Autodesk Inventor part; units mm, degrees
ref_plane "YZ Plane" through (0, 0, 0) normal (1, 0, 0) x (0, 1, 0)
ref_plane "XZ Plane" through (0, 0, 0) normal (0, 1, 0) x (-1, 0, 0)
ref_plane "XY Plane" through (0, 0, 0) normal (0, 0, 1) x (1, 0, 0)
sketch "Szkic1" plane through (0, 0, 0) normal (0, 0, 1) x (1, 0, 0)
  line L0 (-10.5, 0) -> (0, 0)
  line L1 (0, 2) -> (-10.5, 2)
  line L2 (0, 2) -> (-5.359, -18)
  line L3 (-3.8837, -4.7669) -> (-2.0706, 2)
  line L4 (-3.8837, -4.7669) -> (-7.4295, -18)
  line L5 (-7.4295, -18) -> (-5.359, -18)
  dimension "d0" = 2
  dimension "d1" = 75
  dimension "d3" = 2
  dimension "d4" = 20
extrude "Wyciągnięcie proste1" add sketch "Szkic1" against normal blind 50
sketch "Szkic2" plane through (-5.359, -18, 0) normal (0.9659, -0.2588, 0) x (0, 0, -1)
  line L0 (42.7, 8.2894) -> (42.7, 10.6894)
  line L1 (38.3, 8.2894) -> (42.7, 8.2894)
  line L2 (7.3, 8.2894) -> (11.7, 8.2894)
  line L3 (11.7, 8.2894) -> (11.7, 10.6894)
  line L4 (42.7, 8.2894) -> (38.3, 8.2894)
  line L5 (38.3, 8.2894) -> (38.3, 10.6894)
  line L6 (38.3, 10.6894) -> (42.7, 10.6894)
  line L7 (42.7, 10.6894) -> (42.7, 8.2894)
  line L8 (11.7, 8.2894) -> (7.3, 8.2894)
  line L9 (7.3, 8.2894) -> (7.3, 10.6894)
  line L10 (7.3, 10.6894) -> (11.7, 10.6894)
  line L11 (11.7, 10.6894) -> (11.7, 8.2894)
  line L12 (43.7, 11.6894) -> (37.3, 11.6894)
  line L13 (37.3, 11.6894) -> (37.3, 7.2894)
  line L14 (37.3, 7.2894) -> (43.7, 7.2894)
  line L15 (43.7, 7.2894) -> (43.7, 11.6894)
  line L16 (12.7, 11.6894) -> (6.3, 11.6894)
  line L17 (6.3, 11.6894) -> (6.3, 7.2894)
  line L18 (6.3, 7.2894) -> (12.7, 7.2894)
  line L19 (12.7, 7.2894) -> (12.7, 11.6894)
  point P0 (0, 18.7737)
  dimension "d7" = 1
  dimension "d8" = 1
extrude "Wyciągnięcie proste2" cut sketch "Szkic2" against normal through all contours L1 L5 L6 L0 | L9 L10 L3 L2 | L15 L14 L13 L12 | L19 L18 L17 L16
sketch "Szkic3" plane through (0, 0, 0) normal (0, 0, 1) x (1, 0, 0)
  line L0 (-2.0706, 2) -> (-7.4295, -18)
  line L1 (-7.4295, -18) -> (-5.359, -18)
  line L2 (-5.359, -18) -> (0, 2)
  line L3 (0, 2) -> (-2.0706, 2)
  line L4 (-30.5, -19.37) -> (-8.3143, -19.37)
  line L5 (-7.4295, -18) -> (-8.3143, -19.37)
  line L6 (-8.3143, -19.37) -> (-5.7261, -19.37)
  line L7 (-5.7261, -19.37) -> (-5.359, -18)
  point P0 (0, 0)
extrude "Wyciągnięcie proste3" add sketch "Szkic3" against normal up to surface (50 mm away) contours L1 L7 L6 L5
sketch "Szkic4" plane through (0, 0, -50) normal (0, 0, -1) x (-1, 0, 0)
  line L0 (6.5775, -14.82) -> (7.7966, -19.37)
  line L1 (30.5, -19.37) -> (8.3143, -19.37)
  line L2 (8.3143, -19.37) -> (5.7261, -19.37)
  line L3 (7.4295, -18) -> (8.3143, -19.37)
  point P0 (0, 0)
extrude "Wyciągnięcie proste4" cut sketch "Szkic4" against normal through all
sketch "Szkic5" plane through (0, 2, 0) normal (0.9659, -0.2588, 0) x (0, 0, -1)
  circle A0 centre (46.85, -9.9328) radius 1
  circle A1 centre (30.45, -9.9328) radius 1
  circle A2 centre (15.25, -9.9328) radius 1
  point P0 (0, -1.9319)
hole "Otwór1" at (-2.5708, -7.5943, -46.85) at (-2.5708, -7.5943, -15.25) direction (-0.9659, 0.2588, 0) diameter 2.2 depth 2 countersink diameter 4 countersink angle 90
properties part number "noz2"
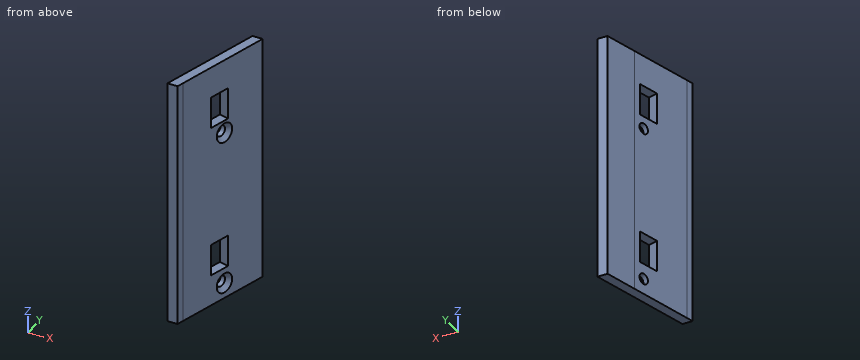
Geometry: final body of the model. Coordinates: model frame, mm. Coordinates: 2 decimals unless noted, no trailing zeros. Write each loop counter-clockwise with the first axis right and the second up, starting at its lowest first coordinate (ties: lowest second). Pieces come first, ordered by that corner, then holes. Notation, with made-up numbers: (58, 0) - (108, 0) arc R8 ccw to (108, 7) - close; hole circle Ø9 at (-8.5, 39). An arc over 180 degrees is marked (long way). Return JSON: item names as keys, results as strings.
Item 1: Line query: L1, parallel to X at y = -18, z = -38.5; L2, parallel to Z at x = -2.75, y = -8; L3, parallel to X at y = -6.25, z = -36.5. Output: solid intervals per line, ascending.
Completed:
{"L1": "x = -7.43 to -5.36", "L2": "z = -50 to -48.73, -44.97 to -43.7, -37.3 to -17.13, -13.37 to -12.7, -6.3 to 0", "L3": "x = -4.28 to -2.21"}
Item 2: Pin query (flat end, axial travel): pin 1 Ø4 at (y, z) = (-14, -18.5) entering from -X; pin 2 Ø12 at (y, z) = (-5.5, -19) entering from +X; pin 3 Ø8 at (y, z) = (-2, -42.5) entering from -X. Return the tip coordinate at first contact, or that it passes through.
Completed:
{"pin 1": "stops at x = -6.89", "pin 2": "stops at x = -0.4", "pin 3": "stops at x = -4.21"}
Item 3: Section query C-C (y = -3.5). Output: boundary loops of the cut face in (x, z).
Completed:
{"outline": "(-3.54, -50) - (-1.47, -50) - (-1.47, 0) - (-3.54, 0) - close"}
Item 4: Section query B-B (x = -6.25). Output: boundary loops of the cut face in (y, z).
Completed:
{"outline": "(-19.37, -50) - (-13.6, -50) - (-13.6, 0) - (-19.37, 0) - close"}
Item 5: Section query A-A (z = -22). Output: boundary loops of the cut face in (x, y), and give its area (3 significant figures).
Completed:
{"outline": "(-7.8, -19.37) - (-5.73, -19.37) - (-5.36, -18) - (0, 2) - (-2.07, 2) - (-3.88, -4.77) - (-7.43, -18) - close", "area": "44.2 mm2"}
